Geometry: final body of the model. Coordinates: model frame, mm. A direction names the side the tool comes from. Round coordinates to 2 decimals unless told otherwise and drop trailing zeros. Loops run counter-clockwise (first coordinate to the right, second up) from the corner with the lowest first, then second, coordinate; pieces in that order, holes last. Notation, with made-up numbers: M 76,52 L 118,52 A25 ccw 118,66 Z; hole C 20.25,-34 d7. An arc over 180 degrees is marked long. Answer as a JSON object with one key per item and string values.
Autodesk Inventor part; units mm, degrees
ref_plane "YZ Plane" through (0, 0, 0) normal (1, 0, 0) x (0, 1, 0)
ref_plane "XZ Plane" through (0, 0, 0) normal (0, 1, 0) x (-1, 0, 0)
ref_plane "XY Plane" through (0, 0, 0) normal (0, 0, 1) x (1, 0, 0)
sketch "底面スケッチ" plane through (0, 0, 0) normal (0, 1, 0) x (-1, 0, 0)
  line L0 (2, 0) -> (43, 0)
  line L1 (45, -2) -> (45, -43)
  line L2 (43, -45) -> (2, -45)
  line L3 (0, -43) -> (0, -2)
  arc A0 (45, -2) -> (43, 0) centre (43, -2) ccw
  arc A1 (43, -45) -> (45, -43) centre (43, -43) ccw
  arc A2 (0, -43) -> (2, -45) centre (2, -43) ccw
  arc A3 (2, 0) -> (0, -2) centre (2, -2) ccw
  point P0 (0, 0)
  point P1 (45, -45)
  point P2 (45, 0)
  point P3 (0, -45)
  dimension "d0" = 45
  dimension "d1" = 45
  dimension "d4" = 2
extrude "押し出し1" add sketch "底面スケッチ" along normal blind 4
sketch "スケッチ2" plane through (0, 4, 0) normal (0, 1, 0) x (1, 0, 0)
  line L0 (-42, 1) -> (-3, 1)
  line L1 (-1, 3) -> (-1, 42)
  line L2 (-3, 44) -> (-42, 44)
  line L3 (-44, 42) -> (-44, 3)
  line L4 (-2, 45) -> (-43, 45)
  line L5 (-43, 0) -> (-2, 0)
  line L6 (-45, 43) -> (-45, 2)
  line L7 (0, 2) -> (0, 43)
  arc A0 (-44, 3) -> (-42, 1) centre (-42, 3) ccw
  arc A1 (-3, 1) -> (-1, 3) centre (-3, 3) ccw
  arc A2 (-42, 44) -> (-44, 42) centre (-42, 42) ccw
  arc A3 (-1, 42) -> (-3, 44) centre (-3, 42) ccw
  point P0 (0, 0)
  dimension "d5" = 1
  dimension "d6" = 1
  dimension "d7" = 1
  dimension "d8" = 1
  dimension "d9" = 2
extrude "押し出し2" cut sketch "スケッチ2" against normal blind 2
sketch "スケッチ3" plane through (0, 2, 0) normal (0, 1, 0) x (1, 0, 0)
  line L0 (-3, 1) -> (-42, 1)
  line L1 (-42, 44) -> (-3, 44)
  line L2 (-44, 3) -> (-44, 42)
  line L3 (-27.5, 2.5) -> (-26, 2.5)
  line L4 (-26, 2.5) -> (-26, 42.5)
  line L5 (-26, 42.5) -> (-27.5, 42.5)
  line L6 (-27.5, 42.5) -> (-27.5, 2.5)
  line L7 (-1, 42) -> (-1, 3)
  line L8 (-27.5, 21.75) -> (-42.5, 21.75)
  line L9 (-42.5, 21.75) -> (-42.5, 23.25)
  line L10 (-42.5, 23.25) -> (-27.5, 23.25)
  line L11 (-27.5, 23.25) -> (-27.5, 21.75)
  point P0 (0, 0)
  point P1 (-26, 22.5)
  point P2 (-1, 22.5)
  point P3 (-42.5, 22.5)
  point P4 (-1, 22.5)
  dimension "d19" = 1.5
  dimension "d20" = 40
  dimension "d21" = 16.5
  dimension "d22" = 1.5
  dimension "d23" = 15
extrude "押し出し3" add sketch "スケッチ3" along normal blind 2
fillet "フィレット1" radius 0.5 3 edges at (-26.75, 4, -42.5) (-26.75, 4, -2.5) (-42.5, 4, -22.5)
fillet "フィレット2" radius 1 8 edges at (-44.4142, 0, -44.4142) (-45, 0, -22.5) (-44.4142, 0, -0.5858) (-22.5, 0, 0) (-0.5858, 0, -0.5858) (0, 0, -22.5) (-0.5858, 0, -44.4142) (-22.5, 0, -45)
sketch "スケッチ4" plane through (0, 4, 0) normal (0, 1, 0) x (1, 0, 0)
  line L0 (-1, 42) -> (-1, 3)
  line L1 (-1, 27.5) -> (0, 27.5)
  line L2 (0, 27.5) -> (0, 17.5)
  line L3 (0, 17.5) -> (-1, 17.5)
  line L4 (-1, 17.5) -> (-1, 27.5)
  line L5 (0, 2) -> (0, 43)
  line L6 (-45, 2) -> (-45, 43)
  line L7 (-44, 43) -> (-44, 2)
  line L8 (-45, 27.5) -> (-44, 27.5)
  line L9 (-44, 27.5) -> (-44, 17.5)
  line L10 (-44, 17.5) -> (-45, 17.5)
  line L11 (-45, 17.5) -> (-45, 27.5)
  point P0 (0, 0)
  point P1 (0, 22.5)
  point P2 (0, 22.5)
  point P3 (-45, 22.5)
  point P4 (-44, 22.5)
  dimension "d24" = 10
  dimension "d25" = 10
extrude "押し出し4" cut sketch "スケッチ4" against normal blind 1.5
fillet "フィレット3" radius 1.5 4 edges at (-44.5, 2.5, -27.5) (-44.5, 2.5, -17.5) (-0.5, 2.5, -27.5) (-0.5, 2.5, -17.5)
fillet "フィレット4" radius 1 8 edges at (-0.5, 3.9995, -27.5) (-0.5, 4, -27.5) (-0.5, 3.9995, -17.5) (-0.5, 4, -17.5) (-44.5, 4, -27.5) (-44.5, 3.9995, -27.5) (-44.5, 4, -17.5) (-44.5, 3.9995, -17.5)
equation "\"d1\" = d0"
equation "\"d6\" = d5"
equation "\"d7\" = d5"
equation "\"d8\" = d5"
equation "\"d25\" = d24"
properties part number "box-2_3D プリント"
1) Pin query (flat end, axial travel): P1, Ø8, axis at x = -16, z = -35.5, coming from the +Y side; P2, Ø1.1, axis at x = -0.5, z = -21, coming from the +Y side. Return the tip coordinate at first contact, or that it passes through.
Results:
{"P1": "y = 2", "P2": "y = 2.5"}
2) Reachability of faces 1 (the flat face through (-29, 4, -23)), 2 (the flat face through (-35, 3, -23.25)), 3 (the cylindrical face through (-44.507, 2.738, -18.188)) from +Z, -Z, +X, -X, +Y, -Y: full face, straight path, thin tool, end or side. Return the list, or none.
Results:
{"face 1": "+Z, -Z, +X, -X, +Y", "face 2": "+Y", "face 3": "-X, +Y"}
3) Section query C-C (z = -21). Return the cut outline in (x, y).
Results:
{"outline": "M -45,1 A1 ccw -44,0 L -1,0 A1 ccw 0,1 L 0,2.5 L -1,2.5 L -1,2 L -26,2 L -26,4 L -27.5,4 L -27.5,2 L -44,2 L -44,2.5 L -45,2.5 Z"}
4) Section query B-B (x = -25). Return the cut outline in (y, z), and give its area (3 significant figures).
Results:
{"outline": "M 0,-44 A1 ccw 1,-45 L 4,-45 L 4,-44 L 2,-44 L 2,-1 L 4,-1 L 4,0 L 1,0 A1 ccw 0,-1 Z", "area": "93.6 mm2"}
5) Ray query, line 1 (Z direction, x = -42, y = 3.3); line 2 (X direction, y = 2.3, z = -37.5); line 3 (Z direction, x = -7.5, y = 2.6). Return the intervals inside material, ascending.
Results:
{"line 1": "-45 to -44, -23.25 to -21.75, -1 to 0", "line 2": "-45 to -44, -27.5 to -26, -1 to 0", "line 3": "-45 to -44, -1 to 0"}
6) Section query A-A (z = -38.5). Return the cut outline in (x, y).
Results:
{"outline": "M -45,1 A1 ccw -44,0 L -1,0 A1 ccw 0,1 L 0,4 L -1,4 L -1,2 L -26,2 L -26,4 L -27.5,4 L -27.5,2 L -44,2 L -44,4 L -45,4 Z"}
7) Pull-direction query (Z, two-part tool) for faces 4 (the flat face through (-42.5, 3, -22)), 5 (the flat face through (-23, 2, -45)), 6 (the flat face through (-27, 3, -42.5)), 7 (the flat face through (-22.4, 4, -44.7)); classes: +Z half, -Z half, draft (parallel to the pull), parting line (faces both ways), or undercut.
Results:
{"face 4": "undercut", "face 5": "-Z half", "face 6": "undercut", "face 7": "draft"}
